```python
from build123d import *

# Parameters (mm, degrees)
F0_R     = 1
F1_DEPTH = 20
F2_R     = 6.25
F3_DEPTH = 5
F5_R     = 17.5
F6_DEPTH = 55


with BuildPart() as f1:
    # F0 (on Front) → F1 (new body)
    with BuildSketch(Plane.XZ):
        Circle(F0_R)
    extrude(amount=F1_DEPTH)

    # F2 (on Front) → F3 (join)
    with BuildSketch(Plane.XZ):
        Circle(F2_R)
    extrude(amount=-F3_DEPTH)

    # F5 (on offset) → F6 (join)
    with BuildSketch(Plane.XZ.offset(-5)):
        Circle(F5_R)
    extrude(amount=-F6_DEPTH)


solid = f1.part
```
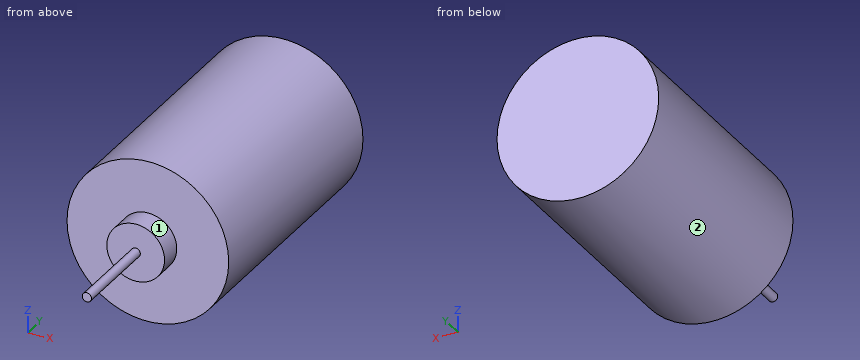
Geometry: final body of the model. Coordinates: model frame, mm. Face numbers are marked on the shaded views. A direction names the side the tool comes from. Round coordinates to 2 decimals unless told otherwise and drop trailing zeros. Order: outer loops, then holes, each group sorted by start corner. A loop starts at its lowest first (then second) coordinate and runs counter-clockwise, first axis right, second up. Notation, with made-up numbers: (-21.75, 79.5) - (-9.75, 79.5) arc R19 cw to (-9.75, 99.5) - close; hole circle Ø9 at (19.5, 21). An arc over 180 degrees is marked (long way). Use CSV: the item, a comma, the result in double quotes. Start each with the question number.
Q1. First-contact query: pin 1 (6 mm diameter, centred on x = 6.5, y = -11.5, fed in from -Z); pin 2 (12 mm diameter, centred on y = 33.5, z = 14, fed in from -X); pin 3 (10 mm diameter, centred on y = 51, z = 1, fed in from -X); pin 4 (4 mm diameter, centred on y = 44, z = 4.5, fed in from +X). Flat tips, straight axial feed; report the tip coordinate or a pass-through.
Q2. Section query B-B (x = 0). Return loops of the section in (y, z), and give its area (3 significant figures).
Q3. Section query C-C (y = 51). Return loops of the section in (x, z), and give its area (3 significant figures).
Q4. Material intervals for line 1 along Y through (x, z) = (-0.5, 9); line 2 along Y through (x, z) = (-3, -1); line 3 along Z through (x, y) = (8, 47.5), sorted ascending. Write a range as from..to.
Q5. Section query D-D (z = -14). Return loops of the section in (x, y).
Q6. Access query for the marked faces 1 and 2. Directions: +Z, -Z, +X, -X, +Y, -Y. A direction counts if a zero-diameter tool reaches every point of the face in a straight line with its end or side. Return the directions, or none.
Q7. Section query A-A (z = 0). Return loops of the section in (x, y), and give its area (3 significant figures).
Result set:
1,pin 1,"passes through"
1,pin 2,"stops at x = -15.56"
1,pin 3,"stops at x = -17.5"
1,pin 4,"stops at x = 17.32"
2,outline,"(-20, -1) - (0, -1) - (0, -6.25) - (5, -6.25) - (5, -17.5) - (60, -17.5) - (60, 17.5) - (5, 17.5) - (5, 6.25) - (0, 6.25) - (0, 1) - (-20, 1) - close"
2,area,"2,030 mm2"
3,outline,"circle Ø35 at (0, 0)"
3,area,"962 mm2"
4,line 1,"y = 5..60"
4,line 2,"y = 0..60"
4,line 3,"z = -15.56..15.56"
5,outline,"(-10.5, 5) - (10.5, 5) - (10.5, 60) - (-10.5, 60) - close"
6,face 1,"-Y"
6,face 2,"+Y, -Y"
7,outline,"(-17.5, 5) - (-6.25, 5) - (-6.25, 0) - (-1, 0) - (-1, -20) - (1, -20) - (1, 0) - (6.25, 0) - (6.25, 5) - (17.5, 5) - (17.5, 60) - (-17.5, 60) - close"
7,area,"2,030 mm2"
